```python
from build123d import *

# Parameters (mm, degrees)
CUT_EXTRUDE1_DEPTH = 1.5
CHAMFER1_SIZE      = 0.2


with BuildPart() as part:
    # Sketch1 → Revolve1 (revolve)
    with BuildSketch(Plane.XY, mode=Mode.PRIVATE) as revolve1_sk:
        Polygon((0, 0), (0, 3), (2, 3), (2, 2), (11.7, 2), (11.7, 0), align=None)
    revolve(revolve1_sk.sketch.rotate(Axis((0, 0, 0), (1, 0, 0)), 180), axis=Axis((0, 0, 0), (1, 0, 0)))

    # Sketch2 → Cut-Extrude1 (cut)
    with BuildSketch(Plane.ZY):
        Polygon((0, 2), (-1.732050808, 1), (-1.732050808, -1), (0, -2), (1.732050808, -1), (1.732050808, 1), align=None)
    extrude(amount=-CUT_EXTRUDE1_DEPTH, mode=Mode.SUBTRACT)

    # Chamfer1
    chamfer1_edges = [part.edges().sort_by_distance(p)[0] for p in [
        (11.7, 2, 0),
        (0, 3, 0),
    ]]
    chamfer(chamfer1_edges, length=CHAMFER1_SIZE)


solid = part.part
```
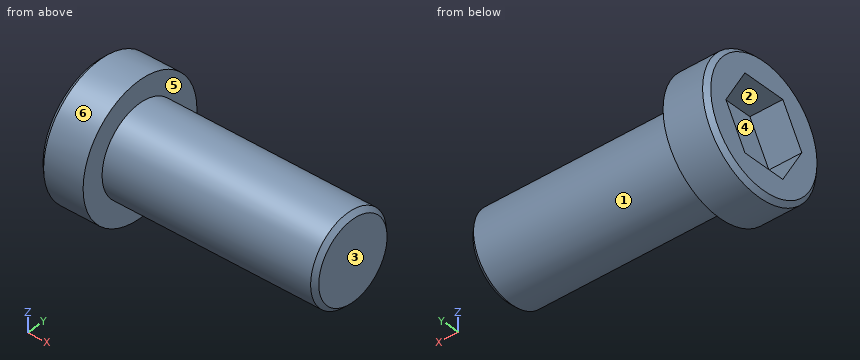
Part model, mm, in its own coordinate system. Face numbers are marked on the shaded views. A direction names the side the tool comes from. Give positions to 0.01 mm unless a question says otherwise; leave off trailing zeros. Loops run counter-clockwise (first coordinate to the right, second up) from the corner with the lowest first, then second, coordinate; pieces in that order, holes last. Notation, with made-up numbers: M 33,77.5 L 91,77.5 A16 cw 91,102.5 Z; hole C -18,49.25 d3. An arc over 180 degrees is marked long. Return JSON: item names as keys, results as strings.
1) 3-axis set-ups, long thin cutter, end or side, ignore diameter. For the marked faces 1, 2 and 3: which of +Z, -Z, +X, -X, +Y, -Y reach the whole face in a straight line?
Calculated:
{"face 1": "+X", "face 2": "-X", "face 3": "+Z, -Z, +X, +Y, -Y"}
2) Saw through at B-B, the plane x = 4.5. List the corners of the cut face in (y, z), then the cut area to 3 significant figures.
Calculated:
{"outline": "C 0,0 d4", "area": "12.6 mm2"}
3) Flat gauge pins, fed straight in: pin 1 Ø2 at (x, y) = (5.5, 0.5) entering from -Z; pin 2 Ø0.8 at (x, y) = (1, -0.5) entering from +Z; pin 3 Ø2 at (x, y) = (6.5, 1.5) entering from +Z; pin 4 Ø1 at (x, z) = (9, -2) entering from +Y. Where does each tip first touch, or does it go through?
Calculated:
{"pin 1": "stops at z = -2", "pin 2": "stops at z = 3", "pin 3": "stops at z = 1.94", "pin 4": "stops at y = 1.32"}
4) Pull direction Y, two halves, no side cores. Call the marked faces 4, 5 and 6: released by +Y, released by -Y, zero draft, split by the parting line, or undercut.
Calculated:
{"face 4": "undercut", "face 5": "zero draft", "face 6": "split by the parting line"}
5) Drill centre lines: line 1 (X direction, y = -0.1, z = 1); line 2 (X direction, y = 0.5, z = -2.1); line 3 (Y direction, x = 1, z = -0.7). Where is each one in solid material? Low to high.
Calculated:
{"line 1": "x = 1.5 to 11.7", "line 2": "x = 0 to 2", "line 3": "y = -2.92 to -1.6, 1.6 to 2.92"}
6) Saw through at A-A, the plane y = 0. List the corners of the cut face in (x, z).
Calculated:
{"outline": "M 0,-2.8 L 0.2,-3 L 2,-3 L 2,-2 L 11.5,-2 L 11.7,-1.8 L 11.7,1.8 L 11.5,2 L 2,2 L 2,3 L 0.2,3 L 0,2.8 L 0,1.73 L 1.5,1.73 L 1.5,-1.73 L 0,-1.73 Z"}
